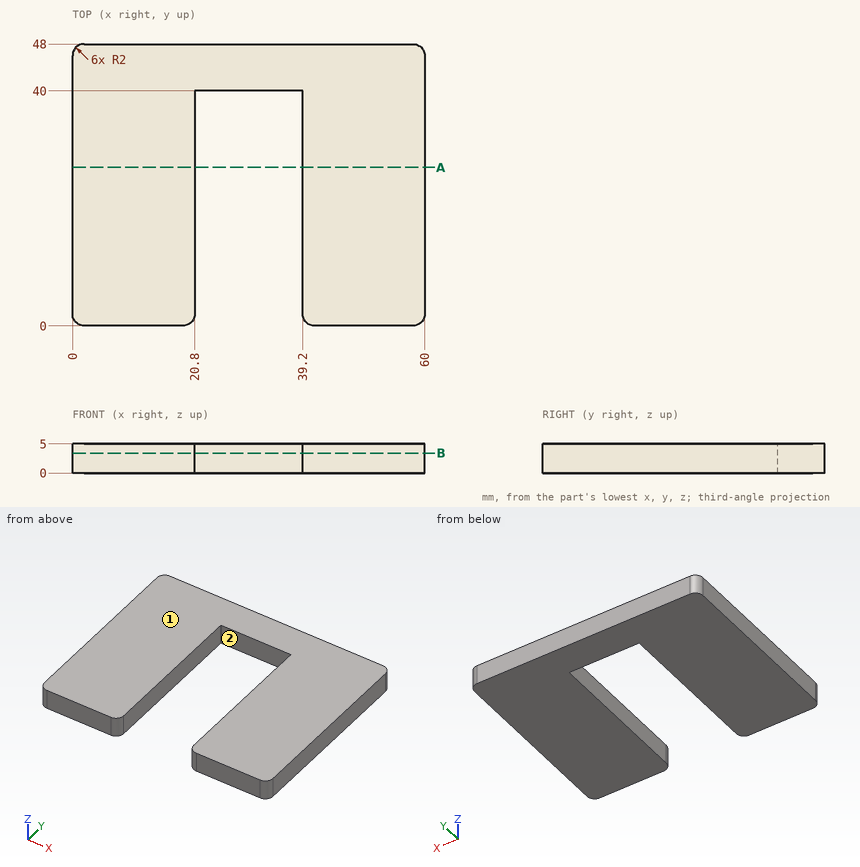
Here's the drawing with two shaded views (mm, measured from the low corner). I have some questions. Give positions to 0.01 mm unless a question says otherwise; leave off trailing zeros. Write each loop counter-clockwise with the first axis right and the second up, starting at its lowest first coordinate (ties: lowest second). Pieces come first, ordered by that corner, then holes. Notation, with made-up numbers: (37.5, 82) -> (65.5, 82) arc R24 cw to (65.5, 101) -> close; hole circle Ø10 at (53.5, -20). An arc over 180 degrees is marked (long way). Answer as a JSON object with one key per item and string values. Group by question number.
Item 1: Suppose I cut it at B-B (z = 3.4). Please give me the cut outline in (x, y).
Item 2: We'd pull the mould along X, two halves only. Please class the marked faces 1 and 2: +X half, -X half, draft (parallel to the pull), parting line (faces both ways), or undercut.
Item 3: Please list where these lines run through material, in increasing order: line 1 (X direction, y = 36.5, z = 2.55); line 2 (Y direction, x = 38, z = 2.5); line 3 (Y direction, x = 20, z = 1.3). Write a range as [from, to].
Item 4: Suppose I cut it at A-A (y = 27). Please give me the cut outline in (x, z).
Findings:
{
 "1": {"outline": "(0, 2) arc R2 ccw to (2, 0) -> (18.8, 0) arc R2 ccw to (20.8, 2) -> (20.8, 40) -> (39.2, 40) -> (39.2, 2) arc R2 ccw to (41.2, 0) -> (58, 0) arc R2 ccw to (60, 2) -> (60, 46) arc R2 ccw to (58, 48) -> (2, 48) arc R2 ccw to (0, 46) -> close"},
 "2": {"face 1": "draft", "face 2": "undercut"},
 "3": {"line 1": "x = [0, 20.8], [39.2, 60]", "line 2": "y = [40, 48]", "line 3": "y = [0.4, 48]"},
 "4": {"outline": "(0, 0) -> (20.8, 0) -> (20.8, 5) -> (0, 5) -> close; (39.2, 0) -> (60, 0) -> (60, 5) -> (39.2, 5) -> close"}
}
